Could you check a few things on this model? Use its own coordinates, in mm. Face numbers are marked on the shaded views. A direction names the side the tool comes from. Give positions to 0.01 mm unless a question says otherwise; leave off trailing zeros. Write each loop counter-clockwise with the first axis right and the second up, starting at its lowest first coordinate (ties: lowest second). Pieces come first, ordered by that corner, then holes. Notation, with made-up numbers: (65, 34) - (100, 34) arc R5 ccw to (100, 43) - close; hole circle Ø7 at (89, 28.25). An arc over 180 degrees is marked (long way). Write item = value, one per line.
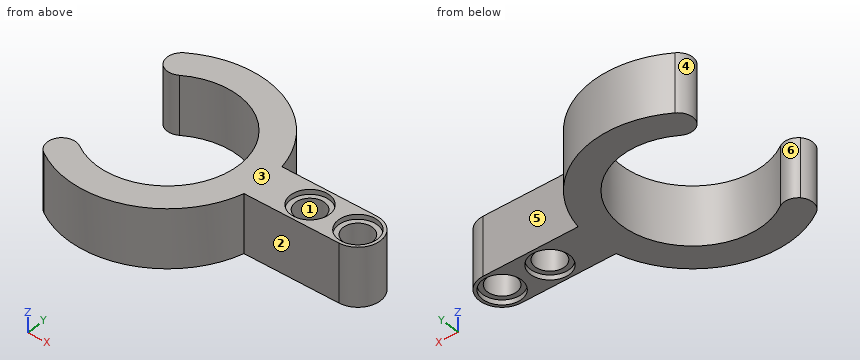
from build123d import *

# Parameters (mm, degrees)
F1_DEPTH    = 9.6
F2_R        = 2.4
F3_DEPTH    = 9.6
F4_T1_DEPTH = 24.0803750693
F4_T3_DEPTH = 20.787199352
F5_R        = 3.2
F6_DEPTH    = 0.8
F7_R        = 3.2
F8_DEPTH    = 0.8


# Not quite as in the source:
# - a fillet or chamfer that OpenCascade refuses, or shapes differently, is made with other operations: its cross-section is extruded or revolved along the edge and cut away or added


with BuildPart() as f1:
    # F0 (on Top) → F1 (new body)
    with BuildSketch(Plane.XY):
        with BuildLine():
            Line((-11.1905737705, 11.9655232935), (-7.9375, 8.4871734989))
            ThreePointArc((-7.9375, 8.4871734989), (11.6205, 0), (-7.9375, -8.4871734989))
            Line((-7.9375, -8.4871734989), (-11.1905737705, -11.9655232935))
            ThreePointArc((-11.1905737705, -11.9655232935), (16.383, 0), (-11.1905737705, 11.9655232935))
        make_face()
    extrude(amount=F1_DEPTH)

    # F2 (on Top) → F3 (join, through all)
    with BuildSketch(Plane.XY):
        with BuildLine():
            Line((31.8347208309, 3.7), (15.9597208309, 3.7))
            ThreePointArc((15.9597208309, 3.7), (16.383, 0), (15.9597208309, -3.7))
            Line((15.9597208309, -3.7), (31.8347208309, -3.7))
            ThreePointArc((31.8347208309, -3.7), (35.5347208309, 0), (31.8347208309, 3.7))
        make_face()
        with Locations((23.8347208309, 0)):
            Circle(F2_R, mode=Mode.SUBTRACT)
        with Locations((31.8347208309, 0)):
            Circle(F2_R, mode=Mode.SUBTRACT)
    extrude(amount=F3_DEPTH)

    # F4: fillet of radius 2.4528409794 on 4 edges, made by hand

    # F4_s2 → F4_t1 (cut)
    with BuildSketch(Plane.XY.offset(-7.2401875346)):
        with BuildLine():
            ThreePointArc((-8.9088227084, 13.7490205815), (-10.0096283387, 11.9889330027), (-9.3664678562, 10.0150976715))
            Line((-9.3664678562, 10.0150976715), (-11.1905737705, 11.9655232935))
            ThreePointArc((-11.1905737705, 11.9655232935), (-10.0891848208, 12.9077898438), (-8.9088227084, 13.7490205815))
        make_face()
        with BuildLine():
            ThreePointArc((-8.9088227084, -13.7490205815), (-10.0096283387, -11.9889330027), (-9.3664678562, -10.0150976715))
            Line((-9.3664678562, -10.0150976715), (-11.1905737705, -11.9655232935))
            ThreePointArc((-11.1905737705, -11.9655232935), (-10.0891848208, -12.9077898438), (-8.9088227084, -13.7490205815))
        make_face()
    extrude(amount=F4_T1_DEPTH, mode=Mode.SUBTRACT)

    # F4_s4 → F4_t3 (cut)
    with BuildSketch(Plane.XY.offset(-5.593599676)):
        with BuildLine():
            ThreePointArc((-9.4658059224, 10.1213149191), (-7.9705260578, 9.3618595516), (-6.3367832056, 9.7406980682))
            ThreePointArc((-6.3367832056, 9.7406980682), (-7.164608937, 9.1490108225), (-7.9375, 8.4871734989))
            Line((-7.9375, 8.4871734989), (-9.4658059224, 10.1213149191))
        make_face()
        with BuildLine():
            ThreePointArc((-9.4658059224, -10.1213149191), (-7.9705260578, -9.3618595516), (-6.3367832056, -9.7406980682))
            ThreePointArc((-6.3367832056, -9.7406980682), (-7.164608937, -9.1490108225), (-7.9375, -8.4871734989))
            Line((-7.9375, -8.4871734989), (-9.4658059224, -10.1213149191))
        make_face()
    extrude(amount=F4_T3_DEPTH, mode=Mode.SUBTRACT)

    # F5 (on face) → F6 (cut)
    with BuildSketch(Plane.XY.offset(9.6)):
        with Locations((23.8347208309, 0)):
            Circle(F5_R)
        with Locations((31.8347208309, 0)):
            Circle(F5_R)
    extrude(amount=-F6_DEPTH, mode=Mode.SUBTRACT)

    # F7 (on face) → F8 (cut)
    with BuildSketch(Plane(origin=(0, 0, 0), x_dir=(1, 0, 0), z_dir=(0, 0, -1))):
        with Locations((23.8347208309, 0)):
            Circle(F7_R)
        with Locations((31.8347208309, 0)):
            Circle(F7_R)
    extrude(amount=-F8_DEPTH, mode=Mode.SUBTRACT)


solid = f1.part
1. Which directions (+Z, -Z, +X, -X, +Y, -Y) give clear straight access to the entire face, cutting with the end or side of a thin tool? Please do the marked faces 4, 5 and 6.
Filled sheet:
face_4 = +Z, -Z, -X
face_5 = +Z, -Z, +X, +Y
face_6 = +Z, -Z
2. If we section it at C-C, the plane z = 3.5: Please give me the cut outline in (x, y) (1 decimal), and give its area (3 significant figures).
Filled sheet:
outline = (-9.4, -10.1) arc R2.5 ccw to (-8.9, -13.7) arc R16.4 ccw to (16, -3.7) - (31.8, -3.7) arc R3.7 ccw to (31.8, 3.7) - (16, 3.7) arc R16.4 ccw to (-8.9, 13.7) arc R2.5 ccw to (-9.4, 10.1) arc R2.5 ccw to (-6.3, 9.7) arc R11.6 cw (long way) to (-6.3, -9.7) arc R2.5 ccw to start; hole circle Ø4.8 at (23.8, 0); hole circle Ø4.8 at (31.8, 0)
area = 405 mm2
3. I need wall thicknesses on line 1 (X direction, y = 0, z = 6.5); line 2 (Y direction, x = 0, z = 7.5); line 3 (Y direction, x = 31, z = 9.25). Which ranges of each line are inside material? Lowest first, please.
Filled sheet:
line_1 = 11.62 to 21.43, 26.23 to 29.43, 34.23 to 35.53
line_2 = -16.38 to -11.62, 11.62 to 16.38
line_3 = -3.7 to -3.09, 3.09 to 3.7
4. If we section it at A-A, the plane y = 0: Please give me the cut outline in (x, z).
Filled sheet:
outline = (11.62, 0) - (20.63, 0) - (20.63, 0.8) - (21.43, 0.8) - (21.43, 8.8) - (20.63, 8.8) - (20.63, 9.6) - (11.62, 9.6) - close; (26.23, 0.8) - (27.03, 0.8) - (27.03, 0) - (28.63, 0) - (28.63, 0.8) - (29.43, 0.8) - (29.43, 8.8) - (28.63, 8.8) - (28.63, 9.6) - (27.03, 9.6) - (27.03, 8.8) - (26.23, 8.8) - close; (34.23, 0.8) - (35.03, 0.8) - (35.03, 0) - (35.53, 0) - (35.53, 9.6) - (35.03, 9.6) - (35.03, 8.8) - (34.23, 8.8) - close
5. Thinking about a two-plate mould opening in Y: for the marked faces 1, 2 and 3, which applies, pulls with the +Y half, pulls with the -Y half, needs draft (parallel to the pull), parting line crosses it, or undercut?
Filled sheet:
face_1 = undercut
face_2 = pulls with the -Y half
face_3 = needs draft
6. If we section it at B-B, the plane x = 0: Please give me the cut outline in (y, z), and give its area (3 significant figures).
Filled sheet:
outline = (-16.38, 0) - (-11.62, 0) - (-11.62, 9.6) - (-16.38, 9.6) - close; (11.62, 0) - (16.38, 0) - (16.38, 9.6) - (11.62, 9.6) - close
area = 91.4 mm2
7. For pin 1 (8.5 mm diameter, centred on x = 31.83, y = 0, fed in from +Z); pin 2 (5 mm diameter, centred on x = 25, z = 7, fed in from +Y); pin 3 (1.9 mm diameter, centred on x = 25.5, y = 1, fed in from -Z); pin 4 (5 mm diameter, centred on x = 24, y = -0.5, fed in from +Z), each with a flat end and sliding along its axis, tell me the tip position at first contact or that it passes through.
Filled sheet:
pin_1 = 9.6
pin_2 = 3.7
pin_3 = 0.8
pin_4 = 8.8
8. If we section it at D-D, the plane x = 9.5: Please give me the cut outline in (y, z), and give its area (3 significant figures).
Filled sheet:
outline = (-13.35, 0) - (-6.69, 0) - (-6.69, 9.6) - (-13.35, 9.6) - close; (6.69, 0) - (13.35, 0) - (13.35, 9.6) - (6.69, 9.6) - close
area = 128 mm2
